from build123d import *

# Parameters (mm, degrees)
F0_W     = 25.4
F0_H     = 31.75
F1_DEPTH = 25.4
F2_W     = 6.633994
F2_H     = 4.925239
F3_DEPTH = 25.401
F5_DEPTH = 25.401
F6_DEPTH = 25.401
F7_DEPTH = 25.401


with BuildPart() as f1:
    # F0 (on Front) → F1 (new body)
    with BuildSketch(Plane.XZ):
        with Locations((12.7, 15.875)):
            Rectangle(F0_W, F0_H)
    extrude(amount=F1_DEPTH)

    # F2 (on face) → F3 (cut, through all)
    with BuildSketch(Plane.XZ.offset(25.4)):
        with Locations((13.06696, 2.462619)):
            Rectangle(F2_W, F2_H)
    extrude(amount=-F3_DEPTH, mode=Mode.SUBTRACT)

    # F4 (on face) → F5 (cut, through all)
    with BuildSketch(Plane.XZ.offset(25.4)):
        Polygon((25.4, 31.75), (0, 31.75), (0, 0), (9.749963, 24.224134), (16.383957, 24.224134), (25.4, 0), align=None)
    extrude(amount=-F5_DEPTH, mode=Mode.SUBTRACT)

    # F2 (on face) → F6 (cut, through all)
    with BuildSketch(Plane.XZ.offset(25.4)):
        Polygon((0, 31.75), (0, 0), (9.749963, 24.224134), (16.383957, 24.224134), (25.4, 0), (25.4, 31.75), align=None)
    extrude(amount=-F6_DEPTH, mode=Mode.SUBTRACT)

    # F2 (on face) → F7 (cut, through all)
    with BuildSketch(Plane.XZ.offset(25.4)):
        Polygon((0, 31.75), (0, 0), (9.749963, 24.224134), (16.383957, 24.224134), (25.4, 0), (25.4, 31.75), align=None)
    extrude(amount=-F7_DEPTH, mode=Mode.SUBTRACT)


solid = f1.part
Read the model definition and answer for the solid it produces. Units are mm, in the model's axes. A direction names the side the tool comes from. Give positions to 0.01 mm unless a question says otherwise; leave off trailing zeros. Write each loop counter-clockwise with the first axis right and the second up, starting at its lowest first coordinate (ties: lowest second). Pieces come first, ordered by that corner, then holes. Notation, with made-up numbers: (-36.75, -15) -> (-9.75, -15) arc R19 cw to (-9.75, -2) -> close; hole circle Ø1 at (23, 82.5). An arc over 180 degrees is marked (long way). Answer as a JSON object with one key per item and string values. Group by question number.
1) The mould has two halves that part along X. Classify faces 1 (the flat face through (13, -13, 4.925)), 2 (the flat face through (20.83, -12.88, 12.28)), 3 (the flat face through (13, -13, 24.224)): +X half, -X half, draft (parallel to the pull), parting line (faces both ways), or undercut.
2) Find section C-C (x = 13). Write down the section's boundary in (y, z).
3) Find section B-B (z = 4.5). Write down the section's boundary in (x, y).
4) A tool of negligible diameter and unlimited length cuts with its end or side. For faces 4 (the flat face through (9.75, -13, 2)), 5 (the flat face through (13, 0, 10)), from which of +Z, -Z, +X, -X, +Y, -Y can it reach the whole face along a straight path? Write none if from no direction.
5) Consider L1, parallel to Z at x = 15.5, y = -20.75; L2, parallel to X at y = -12.5, z = 1.25; L3, parallel to X at y = -20.75, z = 14.5. Determine where each line is inside the solid, lowest interval first. Write a range as from..to.
6) Find section A-A (y = -22). Write down the section's boundary in (x, z), and give its area (3 significant figures).
7) Each of these flat-tipped pins is pushed along its axis until it touches: P1, Ø3, axis at x = 6, y = -21.5, coming from the +Z side; P2, Ø10, axis at y = -14.5, z = 8, coming from the -X side; P3, Ø4, axis at y = -13.5, z = 3.5, coming from the +X side; P4, Ø10, axis at x = 9, y = -15.5, coming from the +Z side. Where does it stop, or does it pass through?
8) Find section D-D (z = 10.25). Write down the section's boundary in (x, y), and give its area (3 significant figures).
Values follow:
{
 "1": {"face 1": "undercut", "face 2": "+X half", "face 3": "draft"},
 "2": {"outline": "(-25.4, 4.93) -> (0, 4.93) -> (0, 24.22) -> (-25.4, 24.22) -> close"},
 "3": {"outline": "(1.81, -25.4) -> (9.75, -25.4) -> (9.75, 0) -> (1.81, 0) -> close; (16.38, -25.4) -> (23.73, -25.4) -> (23.73, 0) -> (16.38, 0) -> close"},
 "4": {"face 4": "-Z, +Y, -Y", "face 5": "+Z, -Z, +X, -X, +Y"},
 "5": {"L1": "z = 4.93..24.22", "L2": "x = 0.5..9.75, 16.38..24.93", "L3": "x = 5.84..20"},
 "6": {"outline": "(0, 0) -> (9.75, 0) -> (9.75, 4.93) -> (16.38, 4.93) -> (16.38, 0) -> (25.4, 0) -> (16.38, 24.22) -> (9.75, 24.22) -> close", "area": "355 mm2"},
 "7": {"P1": "stops at z = 18.63", "P2": "stops at x = 1.21", "P3": "stops at x = 24.84", "P4": "stops at z = 24.22"},
 "8": {"outline": "(4.13, -25.4) -> (21.59, -25.4) -> (21.59, 0) -> (4.13, 0) -> close", "area": "443 mm2"}
}
